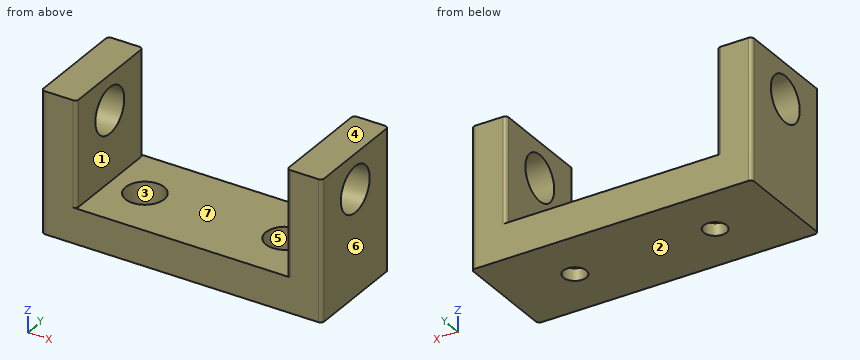
Solid Edge part; units mm, degrees
sketch "Sketch1" plane through (0, 0, 0) normal (0, 0, 1) x (1, 0, 0)
  line L0 (40, -15) -> (40, 15)
  line L1 (40, 15) -> (-40, 15)
  line L2 (-40, 15) -> (-40, -15)
  line L3 (-40, -15) -> (40, -15)
extrude "Protrusion1" add sketch "Sketch1" along normal blind 40
sketch "Sketch2" plane through (0, -15, 20) normal (0, -1, 0) x (1, 0, 0)
  line L0 (-30, -10) -> (-30, 20)
  line L1 (-30, 20) -> (30, 20)
  line L2 (30, 20) -> (30, -10)
  line L3 (30, -10) -> (-30, -10)
extrude "Cutout1" cut sketch "Sketch2" against normal through all
hole "Bohrung_6" at (-20, 0, 10) direction (0, 0, -1) diameter 6.5 end up to next counterbore diameter 11 counterbore depth 6.5
hole "Hole1" at (20, 0, 10) direction (0, 0, -1) diameter 6.5 end up to next counterbore diameter 11 counterbore depth 6.5
hole "Bohrung_8" at (40, 0, 30) direction (-1, 0, 0) diameter 13 end through all
fillet "Verrundung_2" radius 1 8 edges at (-40, -15, 20) (-30, -15, 25) (-30, 15, 25) (-40, 15, 20) (40, -15, 20) (40, 15, 20) (30, -15, 25) (30, 15, 25)
The model under review builds one solid part; all positions refer to its coordinate system, in mm. Face numbers are marked on the shaded views. A direction names the side the tool comes from. Round coordinates to 2 decimals unless told otherwise and drop trailing zeros. Loops run counter-clockwise (first coordinate to the right, second up) from the corner with the lowest first, then second, coordinate; pieces in that order, holes last. Notation, with made-up numbers: (40, -15.75) - (85, -15.75) arc R21 ccw to (85, -3.75) - close; hole circle Ø3 at (-19, 9.5). An arc over 180 degrees is marked (long way). Use a Markdown table: item, result. Add a question column.
Q1. Machinability: for the marked faces 1, 2 and 3, which of the approach directions +Z, -Z, +X, -X, +Y, -Y give a long, thin tool a straight path to every point of the face, cutting with its end or side? Answer none if there is none.
Q2. For probe 1 along X at (y, z) = (0, 2.1); probe 2 along X at (y, z) = (-4.5, 38); probe 3 along X at (y, z) = (0, 8.5), list the stretches that pass through material, from the lowest coordinate up.
Q3. Add section D-D (z = 5). State the section outline as (x, y) points.
Q4. Add section B-B (z = 30). State the section outline as (x, y) points, plus the area to 3 significant figures.
Q5. Add section C-C (y = 0). State how many separate pieces and enclosed holes the cut face has, plus the area to 4 significant figures.
Q6. Insertion check: pin 1 Ø8 at (y, z) = (0, 30) entering from -X; pin 2 Ø12 at (x, y) = (-19.5, -7.5) entering from +Z; pin 3 Ø3.5 at (x, y) = (-22.5, 0) entering from +Z. Each pin has a flat end and moves straight along its axis. Give the tip position at first contact, or say it passes through.
Q7. Add section A-A (x = -20). State the section outline as (y, z) points, plus the area to 3 significant figures.
Q8. The part is to be moulded in two halves that separate along X. For the marked faces 4, 5, 6 and 7, say which applies: pulls with the +X half, pulls with the -X half, needs draft (parallel to the pull), parting line crosses it, or undercut.
Worked answers:
| question | item | result |
|---|---|---|
| 1 | face 1 | +Z, +Y, -Y |
| 1 | face 2 | -Z, +X, -X, +Y, -Y |
| 1 | face 3 | +Z |
| 2 | probe 1 | -40 to -23.25, -16.75 to 16.75, 23.25 to 40 |
| 2 | probe 2 | -40 to -30, 30 to 40 |
| 2 | probe 3 | -40 to -25.5, -14.5 to 14.5, 25.5 to 40 |
| 3 | outline | (-40, -14) arc R1 ccw to (-39, -15) - (39, -15) arc R1 ccw to (40, -14) - (40, 14) arc R1 ccw to (39, 15) - (-39, 15) arc R1 ccw to (-40, 14) - close; hole circle Ø11 at (-20, 0); hole circle Ø11 at (20, 0) |
| 4 | outline | (-40, -14) arc R1 ccw to (-39, -15) - (-31, -15) arc R1 ccw to (-30, -14) - (-30, -6.5) - (-40, -6.5) - close; (-40, 6.5) - (-30, 6.5) - (-30, 14) arc R1 ccw to (-31, 15) - (-39, 15) arc R1 ccw to (-40, 14) - close; (30, -14) arc R1 ccw to (31, -15) - (39, -15) arc R1 ccw to (40, -14) - (40, -6.5) - (30, -6.5) - close; (30, 6.5) - (40, 6.5) - (40, 14) arc R1 ccw to (39, 15) - (31, 15) arc R1 ccw to (30, 14) - close |
| 4 | area | 338 mm² |
| 5 | separate pieces | 5 |
| 5 | enclosed holes | 0 |
| 5 | area | 951.5 mm² |
| 6 | pin 1 | through |
| 6 | pin 2 | z = 10 |
| 6 | pin 3 | z = 3.5 |
| 7 | outline | (-15, 0) - (-3.25, 0) - (-3.25, 3.5) - (-5.5, 3.5) - (-5.5, 10) - (-15, 10) - close; (3.25, 0) - (15, 0) - (15, 10) - (5.5, 10) - (5.5, 3.5) - (3.25, 3.5) - close |
| 7 | area | 206 mm² |
| 8 | face 4 | needs draft |
| 8 | face 5 | undercut |
| 8 | face 6 | pulls with the +X half |
| 8 | face 7 | undercut |
